from build123d import *

# Parameters (mm, degrees)
F0_R      = 15
F0_R_2    = 10
F2_DEPTH  = 10
F1_W      = 6
F1_H      = 2.5
F7_COUNT  = 6
F0_R_3    = 5.25
F0_R_4    = 4
F9_DEPTH  = 4
F10_DEPTH = 9
F11_R     = 0.99999


# Not quite as in the source:
# - a fillet or chamfer is up to 0.001 mm smaller than in the source, because OpenCascade refuses the exact size


with BuildPart() as f2:
    # F0 (on Top) → F2 (new body)
    with BuildSketch(Plane.XY):
        Circle(F0_R)
        Circle(F0_R_2, mode=Mode.SUBTRACT)
    extrude(amount=F2_DEPTH)

    # F6: sweep along a path in F5
    with BuildLine(Plane.YZ.offset(-12)) as f6_path:
        Line((-1.25, 0), (1.4294919243, 10))
    # F1 (on Top) → F6 (sweep)
    with BuildSketch(Plane.XY):
        Polygon((-18, -1.25), (-18, 1.25), (-18, 3), (-20.5, 3), (-20.5, -3), (-18, -3), align=None)
        with Locations((-15, 0)):
            Rectangle(F1_W, F1_H)
    sweep(path=f6_path.line)

    # F7: F2 ×6 about axis
    f7_axis = Axis((0, 0, 0), (0, 0, 1))


with BuildPart() as f2_1:
    add(f2.part)
    for i in range(1, F7_COUNT):
        add(f2.part.rotate(f7_axis, i * 360 / F7_COUNT))



with BuildPart() as f9:
    # F0 (on Top) → F9 (new body)
    with BuildSketch(Plane.XY):
        Circle(F0_R_3)
        Circle(F0_R_4, mode=Mode.SUBTRACT)
    extrude(amount=F9_DEPTH)


with BuildPart() as f2_2:
    add(f2_1.part)

    add(f9.part)  # F10 merges F9
    # F0 (on Top) → F10 (join)
    with BuildSketch(Plane.XY):
        Circle(F0_R_2)
        Circle(F0_R_3, mode=Mode.SUBTRACT)
    extrude(amount=F10_DEPTH)

    # F11 (radius 1 in the source; OpenCascade refuses exactly that, so slightly less here)
    f11_edges = [f2_2.edges().sort_by_distance(p)[0] for p in [
        (-10, 0, 10),
        (-5.25, 0, 9),
    ]]
    fillet(f11_edges, radius=F11_R)


solid = f2_2.part
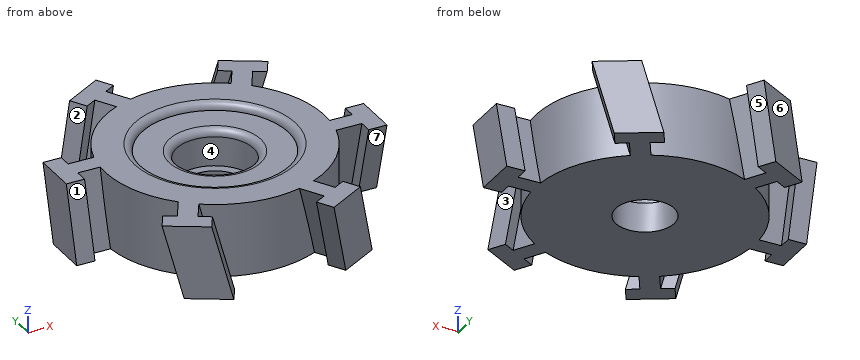
The model under review builds one solid part; all positions refer to its coordinate system, in mm. Face numbers are marked on the shaded views. A direction names the side the tool comes from. Round coordinates to 2 decimals unless told otherwise and drop trailing zeros. Loops run counter-clockwise (first coordinate to the right, second up) from the corner with the lowest first, then second, coordinate; pieces in that order, holes last. Notation, with made-up numbers: (-16.5, 73) -> (12.5, 73) arc R18 cw to (12.5, 102) -> close; hole circle Ø1 at (67.5, 56.5). An arc over 180 degrees is marked (long way). Return JSON: item names as keys, results as strings.
(1) Add section B-B on x = -17. Write out the cut boundary in (y, z), plus the area to 3 significant figures.
Solved:
{"outline": "(-1.25, 0) -> (1.25, 0) -> (3.93, 10) -> (1.43, 10) -> close", "area": "25.0 mm2"}
(2) For pin 1 (1.3 mm diameter, centred on y = 4, z = 3.5, fed in from +X); pin 2 (4 mm diameter, centred on x = 5, z = 1.5, fed in from +Y); pin 3 (8.5 mm diameter, centred on x = 1, y = 2, fed in from +Z), all flat-tipped, find the tip position at first contact; note any pin that passes through.
Solved:
{"pin 1": "x = 14.62", "pin 2": "y = 17.48", "pin 3": "z = 9"}
(3) For the marked faces 1, 2, 3 and 4, list the 3-axis set-ups (+Z, -Z, +X, -X, +Y, -Y) from which the entire face can be reached by the end or side of a thin tool; tool diameter is ignored.
Solved:
{"face 1": "+Z, -X, -Y", "face 2": "+Z, -X", "face 3": "+Z, +X", "face 4": "+Z"}
(4) For line 1 (X direction, y = 0, z = 9.05); line 2 (X direction, y = 0.5, z = 6.75); line 3 (X direction, y = 3.5, z = 3.75), list the stretches that pass through material, from the lowest coordinate up.
Solved:
{"line 1": "-20.5 to -18, -15 to -10, 10 to 15, 18 to 20.5", "line 2": "-20.5 to -18, -14.99 to -5.23, 5.23 to 14.99, 18 to 20.5", "line 3": "-20.5 to -18, -14.59 to -1.94, 1.94 to 14.59"}
(5) The part is to be moulded in two halves that separate along X. For the marked faces 5, 6 and 7, say which applies: released by +X, released by -X, zero draft, split by the parting line, or undercut.
Solved:
{"face 5": "undercut", "face 6": "released by -X", "face 7": "zero draft"}
(6) Add section C-C on y = 2.5. State how many separate pieces and enclosed holes the cut face has, plus the area to 3 significant figures.
Solved:
{"separate pieces": "3", "enclosed holes": "0", "area": "251 mm2"}
